Autodesk Inventor part; units mm, degrees
ref_plane "Work Plane1" through (22, 0, 0) normal (1, 0, 0) x (0, 1, 0)
ref_plane "XZ Plane" through (0, 0, 0) normal (0, 1, 0) x (-1, 0, 0)
ref_plane "XY Plane" through (0, 0, 0) normal (0, 0, 1) x (1, 0, 0)
sketch "Sketch1" plane through (0, 0, 0) normal (0, 0, 1) x (1, 0, 0)
  line L0 (18, -8.5) -> (21, -8.5)
  line L1 (21, -8.5) -> (21, 8.5)
  line L2 (21, 8.5) -> (18, 8.5)
  line L3 (18, 8.5) -> (18, -8.5)
  line L4 (18, -8.5) -> (21, 8.5) construction
  line L5 (21, -8.5) -> (18, 8.5) construction
  line L6 (21, 8.5) -> (22, 8.5)
  line L7 (22, 8.5) -> (22, 5)
  line L8 (22, 5) -> (21, 5)
  line L9 (21, 5) -> (21, 8.5)
  line L10 (21, 1.75) -> (22, 1.75)
  line L11 (22, 1.75) -> (22, -1.75)
  line L12 (22, -1.75) -> (21, -1.75)
  line L13 (21, -1.75) -> (21, 1.75)
  line L14 (21, -5) -> (22, -5)
  line L15 (22, -5) -> (22, -8.5)
  line L16 (22, -8.5) -> (21, -8.5)
  line L17 (21, -8.5) -> (21, -5)
  line L18 (-4.4, 0) -> (26.4, 0)
  line L19 (0, -11.9) -> (0, 11.9)
  point P0 (0, 0)
  point P1 (19.5, 0)
  point P2 (19.5, 0)
  dimension "d2" = 1
  dimension "d3" = 3.5
  dimension "d4" = 8.5
  dimension "d22" = 17
  dimension "d23" = 36
  dimension "d24" = 42
revolve "Revolution1" add sketch "Sketch1" angle 360 about axis through (0, -10, 0) along (0, 1, 0)
sketch "Sketch2" plane through (0, 0, 0) normal (0, 0, 1) x (1, 0, 0)
  line L0 (1, -27.8544) -> (-32.6044, -27.8544)
  line L1 (-32.6044, -27.8544) -> (-32.6044, 28.869)
  line L2 (-32.6044, 28.869) -> (1, 28.869)
  line L3 (1, 28.869) -> (1, -27.8544)
  line L4 (0, -39.1991) -> (0, 40.2136)
  point P0 (0, 0)
  dimension "d8" = 1
extrude "Extrusion1" cut sketch "Sketch2" along normal through all both and the other way through all
ref_plane "Work Plane1" through (22, 0, 0) normal (1, 0, 0) x (0, 1, 0)
sketch "Sketch3" plane through (22, 0, 0) normal (1, 0, 0) x (0, 1, 0)
  point P0 (0, 0)
  point P1 (0, 0)
hole "Hole1" at (22, 0, 0) direction (-1, 0, 0) diameter 2.9 depth 5 counterbore diameter 5.5 counterbore depth 2
chamfer "Chamfer1" distance 0.5 angle 45 6 edges at (15.1538, -1.75, 15.9487) (15.1538, -1.75, -15.9487) (15.1538, 1.75, 15.9487) (15.1538, 1.75, -15.9487) (22, 5, 0) (22, -5, 0)
chamfer "Chamfer2" distance 1 angle 45 2 edges at (22, 8.5, 0) (22, -8.5, 0)
properties part number "Test_Decal_Ring_Tripple"
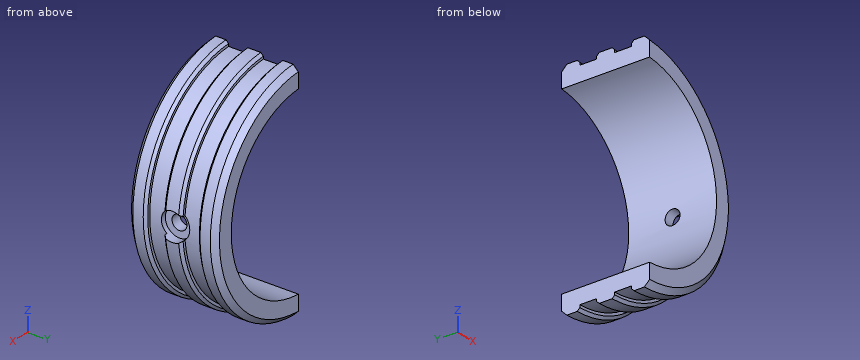
Geometry check sheet. Reference: the model listing, model coordinates, mm. Coordinates: 2 decimals unless noted, no trailing zeros. Order: outer loops, then holes, each group sorted by start corner. A loop starts at its lowest first (then second) coordinate and runs counter-clockwise, first axis right, second up. Notation, with made-up numbers: M 11.25,19.25 L 67.25,19.25 A21 cw 67.25,38.25 Z; hole C -1,45.5 d9. An arc over 180 degrees is marked long. Use CSV: the item, a comma, the result in double quotes.
Item 1: Gauge pin test, flat ends, axial feed: pin 1 Ø5 at (x, y) = (7, -1) entering from -Z; pin 2 Ø2.5 at (y, z) = (0, 0) entering from +X; pin 3 Ø10 at (x, y) = (8, 2) entering from +Z; pin 4 Ø9 at (y, z) = (0, 0) entering from +X. Record the tip position at first contact, or that the pin passes through.
Returned:
pin 1,"stops at z = -21.53"
pin 2,"passes through"
pin 3,"stops at z = 21.79"
pin 4,"stops at x = 21.86"
Item 2: Cross-section at A-A on z = 0. Record the cut outline in (x, y).
Returned:
outline,"M 18,-8.5 L 21,-8.5 L 22,-7.5 L 22,-5.5 L 21.5,-5 L 21,-5 L 21,-2.75 L 20,-2.75 L 20,-1.45 L 18,-1.45 Z; M 18,1.45 L 20,1.45 L 20,2.75 L 21,2.75 L 21,5 L 21.5,5 L 22,5.5 L 22,7.5 L 21,8.5 L 18,8.5 Z"
Item 3: Thickness scan on line 1 along Z through (x, y) = (4.5, 3.5); line 2 along X through (y, z) = (0.25, 1.5); line 3 along Z through (x, y) = (13.5, -2). Record the ranges inside material, lowest first.
Returned:
line 1,"z = -20.51 to -17.43, 17.43 to 20.51"
line 2,"x = 17.94 to 20"
line 3,"z = -16.09 to -11.91, 11.91 to 16.09"
Item 4: Cross-section at B-B on y = 0.5. Record the cut outline in (x, z).
Returned:
outline,"M 1,-21.98 A22 ccw 21.83,-2.7 L 20,-2.7 L 20,-1.36 L 17.95,-1.36 A18 cw 1,-17.97 Z; M 1,17.97 A18 cw 17.95,1.36 L 20,1.36 L 20,2.7 L 21.83,2.7 A22 ccw 1,21.98 Z"
